from build123d import *

# Parameters (mm, degrees)
F0_R        = 19.84
F1_DEPTH    = 8.86
F2_W        = 8.66
F2_H        = 8.8
F3_DEPTH    = 8.86
F4_W        = 8.86
F4_H        = 4.27
F5_DEPTH    = 32.96
F6_R        = 2.84
F7_DEPTH    = 8.86
F8_T1_DEPTH = 8.66
F8_T6_DEPTH = 33.66
F8_S7_R     = 19.84
F8_T8_DEPTH = 19


# Not quite as in the source:
# - a fillet or chamfer that OpenCascade refuses, or shapes differently, is made with other operations: its cross-section is extruded or revolved along the edge and cut away or added


with BuildPart() as f1:
    # F0 (on Top) → F1 (new body)
    with BuildSketch(Plane.XY):
        Circle(F0_R)
    extrude(amount=F1_DEPTH)

    # F2 (on Top) → F3 (join)
    with BuildSketch(Plane.XY):
        with Locations((0, 23.761732877)):
            Rectangle(F2_W, F2_H)
    extrude(amount=F3_DEPTH)

    # F4 (on face) → F5 (join)
    with BuildSketch(Plane.XY.offset(8.86)):
        with Locations((0.1, 26.026732877)):
            Rectangle(F4_W, F4_H)
    extrude(amount=F5_DEPTH)

    # F6 (on face) → F7 (cut, through all)
    with BuildSketch(Plane.XY.offset(8.86)):
        Circle(F6_R)
    extrude(amount=-F7_DEPTH, mode=Mode.SUBTRACT)

    # F8: fillet of radius 5 on 1 edges, made by hand

    # F8_s2 → F8_t1 (join)
    with BuildSketch(Plane.YZ.offset(-4.33)):
        with BuildLine():
            ThreePointArc((18.891732877, 8.86), (22.4272667829, 10.3244660941), (23.891732877, 13.86))
            Line((23.891732877, 13.86), (23.891732877, 8.86))
            Line((23.891732877, 8.86), (18.891732877, 8.86))
        make_face()
    extrude(amount=F8_T1_DEPTH)


with BuildPart() as f8_tool4:
    # F8_s5 → F8_t6 (new body)
    with BuildSketch(Plane.YZ.offset(-16.83)):
        with BuildLine():
            ThreePointArc((18.891732877, 8.86), (22.4272667829, 10.3244660941), (23.891732877, 13.86))
            Line((23.891732877, 13.86), (23.891732877, 8.86))
            Line((23.891732877, 8.86), (18.891732877, 8.86))
        make_face()
    extrude(amount=F8_T6_DEPTH)

    # F8_s7 → F8_t8 (intersect, symmetric)
    with BuildSketch(Plane.XY.offset(11.4)):
        Circle(F8_S7_R)
    extrude(amount=F8_T8_DEPTH, both=True, mode=Mode.INTERSECT)


with BuildPart() as f1_1:
    add(f1.part)

    # F8_t3: union F8_tool4
    add(f8_tool4.part)


solid = f1_1.part
Source: CAD feature listing. Evaluate the final solid. Frame: model axes, mm. A direction names the side the tool comes from. Give positions to 0.01 mm unless a question says otherwise; leave off trailing zeros. Order: outer loops, then holes, each group sorted by start corner. A loop starts at its lowest first (then second) coordinate and runs counter-clockwise, first axis right, second up. Notation, with made-up numbers: (81, 18.5) -> (86, 18.5) arc R19 ccw to (86, 35.5) -> close; hole circle Ø3 at (17, 17.25). An arc over 180 degrees is marked (long way). Use a Markdown table: item, result.
1) Mould query, pull axis Y, two halves, no side actions, for faces 3 (the flat face through (-4.33, 25, 17)), 4 (the cylindrical face through (-2.837, 0.125, 4.492)), 5 (the flat face through (0, 28.162, 21)). Classes: +Y half, -Y half, draft (parallel to the pull), parting line (faces both ways), or undercut.
Answer list:
| item | result |
|---|---|
| face 3 | draft |
| face 4 | undercut |
| face 5 | +Y half |
2) Section query A-A, the plane y = 0. Return the cut outline in (x, z).
Answer list:
| item | result |
|---|---|
| outline | (-19.84, 0) -> (-2.84, 0) -> (-2.84, 8.86) -> (-19.84, 8.86) -> close; (2.84, 0) -> (19.84, 0) -> (19.84, 8.86) -> (2.84, 8.86) -> close |
3) Section query B-B, the plane x = 0. Return the cut outline in (y, z), then the cut area to 3 significant figures.
Answer list:
| item | result |
|---|---|
| outline | (-19.84, 0) -> (-2.84, 0) -> (-2.84, 8.86) -> (-19.84, 8.86) -> close; (2.84, 0) -> (28.16, 0) -> (28.16, 41.82) -> (23.89, 41.82) -> (23.89, 13.86) arc R5 cw to (18.89, 8.86) -> (2.84, 8.86) -> close |
| area | 521 mm² |
4) Reachability of faces 1 (the flat face through (0, 4, 0)), 2 (the flat face through (4, 0, 8.86)) from +Z, -Z, +X, -X, +Y, -Y: full face, straight path, thin tool, end or side. Return the list, or none.
Answer list:
| item | result |
|---|---|
| face 1 | -Z, +X, -X, +Y, -Y |
| face 2 | +Z, +X, -X, -Y |
5) Ray query, line 1 along Y through (x, z) = (0, 6.75); line 2 along Z through (x, y) = (-15, 12.5); line 3 along Y through (x, z) = (-2.5, 18). Return the intervals inside material, ascending. Write a range as [from, to].
Answer list:
| item | result |
|---|---|
| line 1 | [-19.84, -2.84], [2.84, 28.16] |
| line 2 | [0, 8.86] |
| line 3 | [23.89, 28.16] |
6) Contact query for flat-ended pins moving along their axis: P1, Ø3, axis at x = -9.5, y = 14, coming from the +Z side; P2, Ø3, axis at x = 9, z = 8, coming from the +Y side; P3, Ø10, axis at x = -7, y = 22.5, coming from the +Z side; P4, Ø7, axis at y = 24, z = 22, coming from the -X side. Output: stop coordinate, or through.
Answer list:
| item | result |
|---|---|
| P1 | z = 8.86 |
| P2 | y = 18.37 |
| P3 | z = 41.82 |
| P4 | x = -4.33 |
7) Section query C-C, the plane z = 31.5. Return the cut outline in (x, y).
Answer list:
| item | result |
|---|---|
| outline | (-4.33, 23.89) -> (4.53, 23.89) -> (4.53, 28.16) -> (-4.33, 28.16) -> close |
8) Section query D-D, the plane y = -8. Return the cut outline in (x, z), then the cut area to 3 significant figures.
Answer list:
| item | result |
|---|---|
| outline | (-18.16, 0) -> (18.16, 0) -> (18.16, 8.86) -> (-18.16, 8.86) -> close |
| area | 322 mm² |
